Verification items for the finished model (mm, model axes). A direction names the side the tool comes from. Round coordinates to 2 decimals unless told otherwise and drop trailing zeros. Write each loop counter-clockwise with the first axis right and the second up, starting at its lowest first coordinate (ties: lowest second). Pieces come first, ordered by that corner, then holes. Notation, with made-up numbers: M 32.5,73 L 43.5,73 A21 ccw 43.5,108 Z; hole C -15.75,35.5 d5. An arc over 180 degrees is marked long. Use a Markdown table: item, result. Add a question column.
from build123d import *

# Parameters (mm, degrees)
EDIT_GLOBAL_VARIABLE_WITH_PCB_DIMENSIONS_W = 69.96
EDIT_GLOBAL_VARIABLE_WITH_PCB_DIMENSIONS_H = 102.98
BOSS_EXTRUDE1_DEPTH                        = 1.5
FILLET1_R                                  = 3
BOSS_EXTRUDE2_DEPTH                        = 91.1374
BOSS_EXTRUDE3_DEPTH                        = 91.1374
BOSS_EXTRUDE4_DEPTH                        = 58.1174
BOSS_EXTRUDE5_DEPTH                        = 58.1174
FILLET2_R                                  = 0.5
SKETCH7_W                                  = 32
SKETCH7_H                                  = 2.853553391
CUT_EXTRUDE1_DEPTH                         = 35.98
CUT_EXTRUDE1_DEPTH_BACK                    = 35.98
SKETCH8_R                                  = 2.75
BOSS_EXTRUDE6_DEPTH                        = 4
SKETCH11_W                                 = 1.5
SKETCH11_H                                 = 7.5002
BOSS_EXTRUDE8_DEPTH                        = 14.29325
BOSS_EXTRUDE9_DEPTH                        = 14.29325
CHAMFER1_SIZE                              = 7.5
SKETCH10_R                                 = 1.27
BOSS_EXTRUDE10_DEPTH                       = 1.8002


with BuildPart() as part:
    # EDIT GLOBAL VARIABLE WITH PCB DIMENSIONS → Boss-Extrude1 (new body)
    with BuildSketch(Plane(origin=(0, 0, 0), x_dir=(1, 0, 0), z_dir=(0, 1, 0))):
        Rectangle(EDIT_GLOBAL_VARIABLE_WITH_PCB_DIMENSIONS_W, EDIT_GLOBAL_VARIABLE_WITH_PCB_DIMENSIONS_H)
    extrude(amount=BOSS_EXTRUDE1_DEPTH)

    # Fillet1
    fillet1_edges = [part.edges().sort_by_distance(p)[0] for p in [
        (34.98, 0.75, 51.49),
        (-34.98, 0.75, 51.49),
        (-34.98, 0.75, -51.49),
        (34.98, 0.75, -51.49),
    ]]
    fillet(fillet1_edges, radius=FILLET1_R)

    # Sketch2 → Boss-Extrude2 (add)
    with BuildSketch(Plane.XY.offset(45.5687)):
        Polygon((33.18, 1.5), (29.058679656, 1.5), (32.119339828, 4.560660172), (33.18, 3.5), (32.18, 2.5), align=None)
    extrude(amount=-BOSS_EXTRUDE2_DEPTH)

    # Sketch3 → Boss-Extrude3 (add)
    with BuildSketch(Plane.XY.offset(45.5687)):
        Polygon((-33.18, 1.5), (-29.058679656, 1.5), (-32.119339828, 4.560660172), (-33.18, 3.5), (-32.18, 2.5), align=None)
    extrude(amount=-BOSS_EXTRUDE3_DEPTH)

    # Sketch4 → Boss-Extrude4 (add)
    with BuildSketch(Plane.ZY.offset(29.0587)):
        Polygon((-49.69, 1.5), (-45.568679656, 1.5), (-48.629339828, 4.560660172), (-49.69, 3.5), (-48.69, 2.5), align=None)
    extrude(amount=-BOSS_EXTRUDE4_DEPTH)

    # Sketch5 → Boss-Extrude5 (add)
    with BuildSketch(Plane.ZY.offset(29.0587)):
        Polygon((45.568679656, 1.5), (49.69, 1.5), (48.69, 2.5), (49.69, 3.5), (48.629339828, 4.560660172), align=None)
    extrude(amount=-BOSS_EXTRUDE5_DEPTH)

    # Fillet2
    fillet2_edges = [part.edges().sort_by_distance(p)[0] for p in [
        (33.18, 3.5, 0),
        (32.119339828, 4.560660172, 0),
        (-32.119339828, 4.560660172, 0),
        (-33.18, 3.5, 0),
        (0, 4.560660172, -48.629339828),
        (0, 3.5, -49.69),
        (0, 3.5, 49.69),
        (0, 4.560660172, 48.629339828),
    ]]
    fillet(fillet2_edges, radius=FILLET2_R)

    # Sketch7 → Cut-Extrude1 (cut, two sides)
    with BuildSketch(Plane(origin=(0, 0, 0), x_dir=(0, 0, -1), z_dir=(1, 0, 0))) as cut_extrude1_sk:
        with Locations((0, 2.926776696)):
            Rectangle(SKETCH7_W, SKETCH7_H)
    extrude(amount=CUT_EXTRUDE1_DEPTH, mode=Mode.SUBTRACT)
    extrude(cut_extrude1_sk.sketch, amount=-CUT_EXTRUDE1_DEPTH_BACK, mode=Mode.SUBTRACT)

    # Sketch8 → Boss-Extrude6 (add)
    with BuildSketch(Plane(origin=(0, 1.5, 0), x_dir=(1, 0, 0), z_dir=(0, 1, 0))):
        with Locations(Location((-26.98732474, 43.49732474, 0), (0, 0, 131.129923219))):  # turned: the seam where the file's is
            Circle(SKETCH8_R)
        with Locations(Location((26.98732474, 43.49732474, 0), (0, 0, 131.129923219))):  # turned: the seam where the file's is
            Circle(SKETCH8_R)
        with Locations(Location((-26.98732474, -43.49732474, 0), (0, 0, 138.870076781))):  # turned: the seam where the file's is
            Circle(SKETCH8_R)
        with Locations(Location((26.98732474, -43.49732474, 0), (0, 0, 41.129923219))):  # turned: the seam where the file's is
            Circle(SKETCH8_R)
    extrude(amount=BOSS_EXTRUDE6_DEPTH)

    # Sketch11 → Boss-Extrude8 (add, symmetric)
    with BuildSketch(Plane.XY):
        with Locations((-31.43, 5.2501)):
            Rectangle(SKETCH11_W, SKETCH11_H)
        with Locations((31.43, 5.2501)):
            Rectangle(SKETCH11_W, SKETCH11_H)
    extrude(amount=BOSS_EXTRUDE8_DEPTH, both=True)

    # Sketch12 → Boss-Extrude9 (add, symmetric)
    with BuildSketch(Plane.XY):
        Polygon((30.68, 9.0002), (30.68, 7.0002), (29.68, 8.0002), align=None)
        Polygon((-30.68, 9.0002), (-30.68, 7.0002), (-29.68, 8.0002), align=None)
    extrude(amount=BOSS_EXTRUDE9_DEPTH, both=True)

    # Chamfer1
    chamfer1_edges = [part.edges().sort_by_distance(p)[0] for p in [
        (31.43, 9.0002, -14.29325),
        (31.43, 9.0002, 14.29325),
        (-31.43, 9.0002, -14.29325),
        (-31.43, 9.0002, 14.29325),
    ]]
    chamfer(chamfer1_edges, length=CHAMFER1_SIZE)

    # Sketch10 → Boss-Extrude10 (add)
    with BuildSketch(Plane(origin=(0, 5.5, 0), x_dir=(1, 0, 0), z_dir=(0, 1, 0))):
        with Locations(Location((-26.98732474, 43.49732474, 0), (0, 0, 270))):  # turned: the seam where the file's is
            Circle(SKETCH10_R)
        with Locations(Location((26.98732474, 43.49732474, 0), (0, 0, 270))):  # turned: the seam where the file's is
            Circle(SKETCH10_R)
        with Locations(Location((26.98732474, -43.49732474, 0), (0, 0, 270))):  # turned: the seam where the file's is
            Circle(SKETCH10_R)
        with Locations(Location((-26.98732474, -43.49732474, 0), (0, 0, 270))):  # turned: the seam where the file's is
            Circle(SKETCH10_R)
    extrude(amount=BOSS_EXTRUDE10_DEPTH)


solid = part.part
1. Release check for a two-part mould opening along X. For faces 4 (the flat face through (-32.18, 4, 0)), 5 (the cylindrical face through (25.169, 3.472, -41.434)), 6 (the flat face through (27, 7.3, 43)) record: +X half, -X half, draft (parallel to the pull), parting line (faces both ways), or undercut.
2. Access from +Z, -Z, +X, -X, +Y, -Y to the whole of each face (thin tool, end or side, straight path). Record for faces 1 (the flat face through (-26, 5.5, -45)), 2 (the flat face through (-32, 3, 16)), 3 (the flat face through (-30.68, 4, 0)).
3. Depth check by flat-ended pin: pin 1 Ø4.5 at (x, z) = (-26, -44.5) entering from +Y; pin 2 Ø2 at (x, y) = (-18, 5.5) entering from +Z; pin 3 Ø2 at (y, z) = (3, 22) entering from -X; pin 4 Ø0.9 at (x, y) = (-32, 3) entering from -Z. Enter the tip coordinate at first touch or a pass-through.
4. Cross-section at C-C on z = -1.5. Enter the section's corners in (x, y), plus the area to 3 significant figures.
5. Cross-section at A-A on x = -12. Enter the section's corners in (y, z).
6. Scan lines: line 1 along X through (y, z) = (3.5, -45.5); line 2 along X through (y, z) = (6.5, 5.5); line 3 along Y through (x, z) = (5, 37). Record each from-to range of solid material in increasing order. Write a range as from..to.
7. Cross-section at B-B on z = -23. Enter the section's corners in (x, y).
Answer:
| question | item | result |
|---|---|---|
| 1 | face 4 | -X half |
| 1 | face 5 | undercut |
| 1 | face 6 | draft |
| 2 | face 1 | +Y |
| 2 | face 2 | +X, -X, +Y |
| 2 | face 3 | none |
| 3 | pin 1 | stops at y = 7.3 |
| 3 | pin 2 | passes through |
| 3 | pin 3 | stops at x = -32.97 |
| 3 | pin 4 | stops at z = -45.57 |
| 4 | outline | M -34.98,0 L 34.98,0 L 34.98,1.5 L 32.18,1.5 L 32.18,9 L 30.68,9 L 29.68,8 L 30.68,7 L 30.68,1.5 L -30.68,1.5 L -30.68,7 L -29.68,8 L -30.68,9 L -32.18,9 L -32.18,1.5 L -34.98,1.5 Z |
| 4 | area | 129 mm^2 |
| 5 | outline | M 0,-51.49 L 1.5,-51.49 L 1.5,-49.69 L 2.5,-48.69 L 3.15,-49.34 A0.5 ccw 3.85,-49.34 L 4.21,-48.98 A0.5 ccw 4.21,-48.28 L 1.5,-45.57 L 1.5,45.57 L 4.21,48.28 A0.5 ccw 4.21,48.98 L 3.85,49.34 A0.5 ccw 3.15,49.34 L 2.5,48.69 L 1.5,49.69 L 1.5,51.49 L 0,51.49 Z |
| 6 | line 1 | x = -32.97..-31.06, -28.87..-25.1, 25.1..28.87, 31.06..32.97 |
| 6 | line 2 | x = -32.18..-30.68, 30.68..32.18 |
| 6 | line 3 | y = 0..1.5 |
| 7 | outline | M -34.98,0 L 34.98,0 L 34.98,1.5 L 33.18,1.5 L 32.18,2.5 L 32.83,3.15 A0.5 ccw 32.83,3.85 L 32.47,4.21 A0.5 ccw 31.77,4.21 L 29.06,1.5 L -29.06,1.5 L -31.77,4.21 A0.5 ccw -32.47,4.21 L -32.83,3.85 A0.5 ccw -32.83,3.15 L -32.18,2.5 L -33.18,1.5 L -34.98,1.5 Z |
